The model under review builds one solid part; all positions refer to its coordinate system, in mm. Face numbers are marked on the shaded views. A direction names the side the tool comes from. Round coordinates to 2 decimals unless told otherwise and drop trailing zeros. Order: outer loops, then holes, each group sorted by start corner. A loop starts at its lowest first (then second) coordinate and runs counter-clockwise, first axis right, second up.
```python
from build123d import *

# Parameters (mm, degrees)
F2_DEPTH  = 15
F1_W      = 885
F1_H      = 570
F3_DEPTH  = 15
F4_W      = 900
F4_H      = 735
F5_DEPTH  = 15
F8_DEPTH  = 15
F10_W     = 870
F10_H     = 720
F11_DEPTH = 15


with BuildPart() as f2:
    # F0 (on Right) → F2 (new body)
    with BuildSketch(Plane.YZ):
        Polygon((0, 735), (0, 0), (15, 0), (15, -140), (570, -140), (570, 0), (570, 735), align=None)
    extrude(amount=F2_DEPTH)

    # F1 (on Top) → F3 (join)
    with BuildSketch(Plane.XY):
        with Locations((442.5, 285)):
            Rectangle(F1_W, F1_H)
    extrude(amount=F3_DEPTH)

    # F4 (on Front) → F5 (join)
    with BuildSketch(Plane.XZ):
        with Locations((450, 367.5)):
            Rectangle(F4_W, F4_H)
    extrude(amount=F5_DEPTH)

    # F7 (on offset) → F8 (join)
    with BuildSketch(Plane.YZ.offset(885)):
        Polygon((0, 735), (0, 0), (15, 0), (15, -140), (570, -140), (570, 735), align=None)
    extrude(amount=F8_DEPTH)

    # F10 (on offset) → F11 (join)
    with BuildSketch(Plane(origin=(0, 504, 0), x_dir=(-1, 0, 0), z_dir=(0, 1, 0))):
        with Locations((-450, 375)):
            Rectangle(F10_W, F10_H)
    extrude(amount=-F11_DEPTH)


solid = f2.part
```
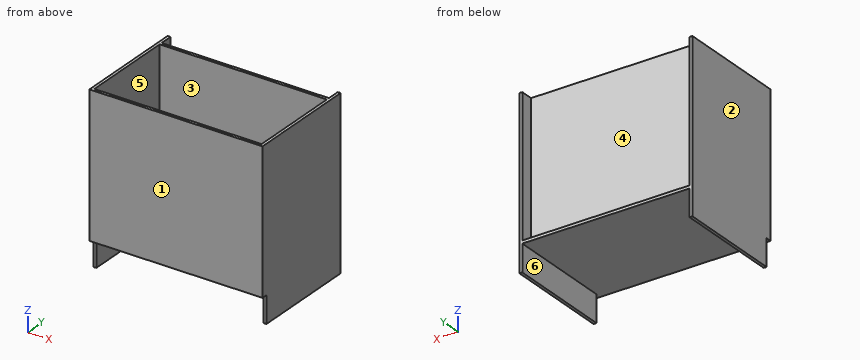
(1) Draft analysis for pull direction X (two halves, no side actions). For the marked faces 1, 2 and 3, state which applies: pulls with the +X half, pulls with the -X half, needs draft (parallel to the pull), parting line crosses it, or undercut.
Data:
face 1: needs draft
face 2: pulls with the -X half
face 3: undercut
(2) For the marked faces 4, 5 and 6, list the 3-axis set-ups (+Z, -Z, +X, -X, +Y, -Y) from which the entire face can be reached by the end or side of a thin tool; tool diameter is ignored.
Data:
face 4: +Z, +Y
face 5: +Z
face 6: -Z, +Y, -Y
(3) Consider section B-B (y = 287.5). Write out the cut boundary in (x, z), and give its area (3 significant figures).
Data:
outline: (0, -140) - (15, -140) - (15, 0) - (885, 0) - (885, -140) - (900, -140) - (900, 735) - (885, 735) - (885, 15) - (15, 15) - (15, 735) - (0, 735) - close
area: 39,300 mm2
(4) Consider section A-A (x = 80). Write out the cut boundary in (y, z).
Data:
outline: (-15, 0) - (570, 0) - (570, 15) - (504, 15) - (504, 735) - (489, 735) - (489, 15) - (0, 15) - (0, 735) - (-15, 735) - close
(5) To check wall thickness, follow probe 1 along X at (y, z) = (253.5, -31); probe 2 along Y at (x, z) = (42, 161); probe 3 along Z at (x, y) = (574, 317). State the ranges of each line that lie inside material, in increasing order.
Data:
probe 1: x = 0 to 15, 885 to 900
probe 2: y = -15 to 0, 489 to 504
probe 3: z = 0 to 15
(6) Consider section C-C (z = 212). Write out the cut boundary in (x, y).
Data:
outline: (0, -15) - (900, -15) - (900, 570) - (885, 570) - (885, 504) - (15, 504) - (15, 570) - (0, 570) - close; hole (15, 0) - (885, 0) - (885, 489) - (15, 489) - close
(7) Insertion check: pin 1 (6 mm diameter, centred on y = 313.5, z = 561, fed in from -X); pin 2 (6 mm diameter, centred on x = 378.5, y = 453, fed in from -Z); pin 3 (7.5 mm diameter, centred on x = 895.5, z = -93.5, fed in from -Y); pin 4 (10 mm diameter, centred on x = 317.5, z = 118.5, fed in from +Y). Each pin has a flat end and moves straight along its axis. Give the tip position at first contact, or say it passes through.
Data:
pin 1: stops at x = 0
pin 2: stops at z = 0
pin 3: stops at y = 15
pin 4: stops at y = 504
